Answer from the drawing. Dimensions are ordinates in mm from the lowest x, y and z of the part. A direction names the side the tool comes from. Give positions to 0.01 mm unless a question says otherwise; leave off trailing zeros. Loops run counter-clockwise (first coordinate to the right, second up) from the corner with the lowest first, then second, coordinate; pieces in that order, holes last. Notation, with made-up numbers: (12, 15) -> (64, 15) arc R26 ccw to (64, 51) -> close; hole circle Ø8 at (-29, 49.5). An arc over 180 degrees is marked (long way). Write each question's results on one line, items separated by ' | '. Start each with the question number.
Item 1: Section A-A on z = 23.5 is taken. Write down the section's boundary in (x, y) (1 decimal).
Item 2: Section B-B on z = 50.5 is taken. Write down the section's boundary in (x, y) (1 decimal).
Item 3: Section C-C on x = 8 is taken. Write down the section's boundary in (y, z) (1 decimal), and give its area (3 significant figures).
Item 4: Each of these flat-tipped pins is pushed along its axis until it touches: P1, Ø1.5, axis at y = 6, z = 80.5, coming from the -X side (1 decimal); P2, Ø5, axis at y = 3, z = 24.5, coming from the -X side; P3, Ø3, axis at y = 5, z = 109.5, coming from the +X side (1 decimal). Where does it stop, or does it pass through?
Item 5: Section D-D on x = 29 is taken. Write down the section's boundary in (y, z) (1 decimal).
Item 6: Which of the six approach directions +Z, -Z, +X, -X, +Y, -Y give full straight-line access (tool end or side, diameter ignored) to the marked faces 1, 2 and 3?
Item 7: Find the intervals of material crossed by line 1 (X direction, y = 1.75, z = 66) (1 decimal); line 2 (X direction, y = 2.5, z = 104) (1 decimal); line 3 (Y direction, x = 34, z = 84), in increasing order.
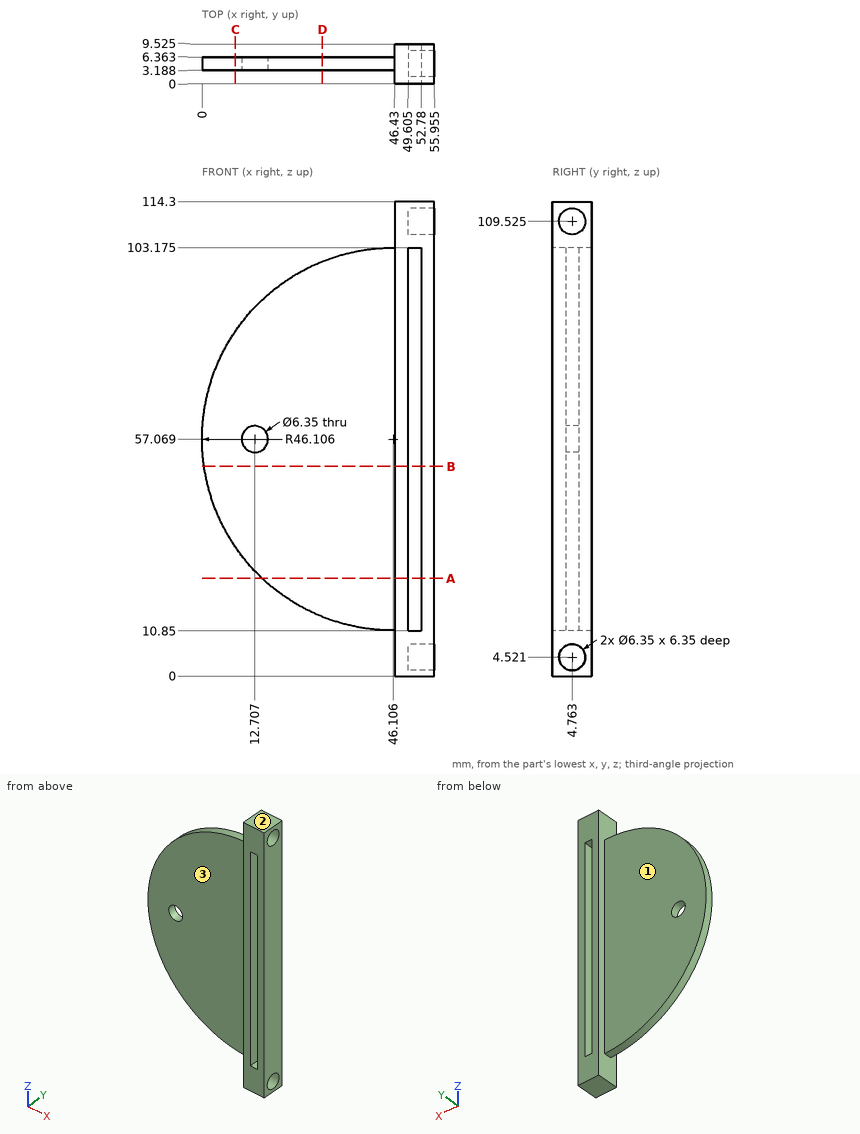
Findings:
1) outline: (14.5, 3.2) -> (46.4, 3.2) -> (46.4, 0) -> (49.6, 0) -> (49.6, 9.5) -> (46.4, 9.5) -> (46.4, 6.4) -> (14.5, 6.4) -> close; (52.8, 0) -> (56, 0) -> (56, 9.5) -> (52.8, 9.5) -> close
2) outline: (0.5, 3.2) -> (46.4, 3.2) -> (46.4, 0) -> (49.6, 0) -> (49.6, 9.5) -> (46.4, 9.5) -> (46.4, 6.4) -> (0.5, 6.4) -> close; (52.8, 0) -> (56, 0) -> (56, 9.5) -> (52.8, 9.5) -> close
3) outline: (3.2, 31.1) -> (6.4, 31.1) -> (6.4, 83) -> (3.2, 83) -> close | area: 165 mm2
4) P1: x = 6 | P2: x = 11.16 | P3: x = 49.6
5) outline: (3.2, 14.3) -> (6.4, 14.3) -> (6.4, 99.9) -> (3.2, 99.9) -> close
6) face 1: +Z, -Z, -X, +Y | face 2: +Z, +X, -X, +Y, -Y | face 3: +Z, -Z, -X, -Y
7) line 1: 46.4 to 49.6, 52.8 to 56 | line 2: 46.4 to 56 | line 3: 3.19 to 6.36
